from build123d import *

# Parameters (mm, degrees)
SKETCH1_W           = 5.08
SKETCH1_H           = 25.4
BOSS_EXTRUDE1_DEPTH = 5.08


with BuildPart() as part:
    # Sketch1 → Boss-Extrude1 (new body)
    with BuildSketch(Plane.XY):
        with BuildLine():
            Line((-13.447242614, 88.667051475), (-13.447242614, 93.747051475))
            Line((-13.447242614, 93.747051475), (9.557461427, 93.747051475))
            ThreePointArc((9.557461427, 93.747051475), (7.2409193, 101.644458486), (2.277698276, 108.209657797))
            Line((2.277698276, 108.209657797), (-45.487793081, 152.041039764))
            ThreePointArc((-45.487793081, 152.041039764), (-50.959133788, 159.684872704), (-52.891849255, 168.884240186))
            Line((-52.891849255, 168.884240186), (-52.891849255, 188.293861482))
            Line((-52.891849255, 188.293861482), (-52.891849255, 199.743466198))
            ThreePointArc((-52.891849255, 199.743466198), (-50.959133788, 208.94283368), (-45.487793081, 216.58666662))
            Line((-45.487793081, 216.58666662), (2.277698276, 260.418048586))
            ThreePointArc((2.277698276, 260.418048586), (7.2409193, 266.983247897), (9.557461427, 274.880654909))
            Line((9.557461427, 274.880654909), (-13.447242614, 274.880654909))
            Line((-13.447242614, 274.880654909), (-13.447242614, 279.960654909))
            Line((-13.447242614, 279.960654909), (-14.800406259, 279.960654909))
            Line((-14.800406259, 279.960654909), (-38.847242614, 279.960654909))
            Line((-38.847242614, 279.960654909), (-38.847242614, 274.880654909))
            Line((-38.847242614, 274.880654909), (-49.891849255, 274.880654909))
            Line((-49.891849255, 274.880654909), (-49.891849255, 264.914705614))
            Line((-49.891849255, 264.914705614), (-47.351849255, 264.914705614))
            Line((-47.351849255, 264.914705614), (-47.351849255, 262.414705614))
            Line((-47.351849255, 262.414705614), (-49.891849255, 262.414705614))
            Line((-49.891849255, 262.414705614), (-49.891849255, 260.680654909))
            Line((-49.891849255, 260.680654909), (-52.891849255, 260.680654909))
            Line((-52.891849255, 260.680654909), (-52.891849255, 262.414705614))
            Line((-52.891849255, 262.414705614), (-55.431849255, 262.414705614))
            Line((-55.431849255, 262.414705614), (-55.431849255, 264.914705614))
            Line((-55.431849255, 264.914705614), (-52.891849255, 264.914705614))
            Line((-52.891849255, 264.914705614), (-52.891849255, 274.880654909))
            Line((-52.891849255, 274.880654909), (-130.862222045, 274.880654909))
            Line((-130.862222045, 274.880654909), (-130.862222045, 264.914705614))
            Line((-130.862222045, 264.914705614), (-128.322222045, 264.914705614))
            Line((-128.322222045, 264.914705614), (-128.322222045, 262.414705614))
            Line((-128.322222045, 262.414705614), (-130.862222045, 262.414705614))
            Line((-130.862222045, 262.414705614), (-130.862222045, 260.680654909))
            Line((-130.862222045, 260.680654909), (-133.862222045, 260.680654909))
            Line((-133.862222045, 260.680654909), (-133.862222045, 262.414705614))
            Line((-133.862222045, 262.414705614), (-136.402222045, 262.414705614))
            Line((-136.402222045, 262.414705614), (-136.402222045, 264.914705614))
            Line((-136.402222045, 264.914705614), (-133.862222045, 264.914705614))
            Line((-133.862222045, 264.914705614), (-133.862222045, 274.880654909))
            Line((-133.862222045, 274.880654909), (-144.906828687, 274.880654909))
            Line((-144.906828687, 274.880654909), (-144.906828687, 279.960654909))
            Line((-144.906828687, 279.960654909), (-168.953665042, 279.960654909))
            Line((-168.953665042, 279.960654909), (-170.306828687, 279.960654909))
            Line((-170.306828687, 279.960654909), (-170.306828687, 274.880654909))
            Line((-170.306828687, 274.880654909), (-193.311532727, 274.880654909))
            ThreePointArc((-193.311532727, 274.880654909), (-190.9949906, 266.983247897), (-186.031769576, 260.418048586))
            Line((-186.031769576, 260.418048586), (-138.266278219, 216.58666662))
            ThreePointArc((-138.266278219, 216.58666662), (-132.794937512, 208.94283368), (-130.862222045, 199.743466198))
            Line((-130.862222045, 199.743466198), (-130.862222045, 188.293861482))
            Line((-130.862222045, 188.293861482), (-130.862222045, 168.884240186))
            ThreePointArc((-130.862222045, 168.884240186), (-132.794937512, 159.684872704), (-138.266278219, 152.041039764))
            Line((-138.266278219, 152.041039764), (-186.031769576, 108.209657797))
            ThreePointArc((-186.031769576, 108.209657797), (-190.9949906, 101.644458486), (-193.311532727, 93.747051475))
            Line((-193.311532727, 93.747051475), (-170.306828687, 93.747051475))
            Line((-170.306828687, 93.747051475), (-170.306828687, 88.667051475))
            Line((-170.306828687, 88.667051475), (-168.953665042, 88.667051475))
            Line((-168.953665042, 88.667051475), (-144.906828687, 88.667051475))
            Line((-144.906828687, 88.667051475), (-144.906828687, 93.747051475))
            Line((-144.906828687, 93.747051475), (-133.862222045, 93.747051475))
            Line((-133.862222045, 93.747051475), (-133.862222045, 103.713000769))
            Line((-133.862222045, 103.713000769), (-136.402222045, 103.713000769))
            Line((-136.402222045, 103.713000769), (-136.402222045, 106.213000769))
            Line((-136.402222045, 106.213000769), (-133.862222045, 106.213000769))
            Line((-133.862222045, 106.213000769), (-133.862222045, 107.947051475))
            Line((-133.862222045, 107.947051475), (-130.862222045, 107.947051475))
            Line((-130.862222045, 107.947051475), (-130.862222045, 106.213000769))
            Line((-130.862222045, 106.213000769), (-128.322222045, 106.213000769))
            Line((-128.322222045, 106.213000769), (-128.322222045, 103.713000769))
            Line((-128.322222045, 103.713000769), (-130.862222045, 103.713000769))
            Line((-130.862222045, 103.713000769), (-130.862222045, 93.747051475))
            Line((-130.862222045, 93.747051475), (-52.891849255, 93.747051475))
            Line((-52.891849255, 93.747051475), (-52.891849255, 103.713000769))
            Line((-52.891849255, 103.713000769), (-55.431849255, 103.713000769))
            Line((-55.431849255, 103.713000769), (-55.431849255, 106.213000769))
            Line((-55.431849255, 106.213000769), (-52.891849255, 106.213000769))
            Line((-52.891849255, 106.213000769), (-52.891849255, 107.947051475))
            Line((-52.891849255, 107.947051475), (-49.891849255, 107.947051475))
            Line((-49.891849255, 107.947051475), (-49.891849255, 106.213000769))
            Line((-49.891849255, 106.213000769), (-47.351849255, 106.213000769))
            Line((-47.351849255, 106.213000769), (-47.351849255, 103.713000769))
            Line((-47.351849255, 103.713000769), (-49.891849255, 103.713000769))
            Line((-49.891849255, 103.713000769), (-49.891849255, 93.747051475))
            Line((-49.891849255, 93.747051475), (-38.847242614, 93.747051475))
            Line((-38.847242614, 93.747051475), (-38.847242614, 88.667051475))
            Line((-38.847242614, 88.667051475), (-14.800406259, 88.667051475))
            Line((-14.800406259, 88.667051475), (-13.447242614, 88.667051475))
        make_face()
        with Locations((-91.87703565, 142.791515907)):
            Rectangle(SKETCH1_W, SKETCH1_H, mode=Mode.SUBTRACT)
        with Locations((-91.87703565, 233.796207057)):
            Rectangle(SKETCH1_W, SKETCH1_H, mode=Mode.SUBTRACT)
    extrude(amount=BOSS_EXTRUDE1_DEPTH)


solid = part.part
Check sheet for the modelled part. Datum: model origin and axes. Units: mm. A direction names the side the tool comes from. Give positions to 0.01 mm unless a question says otherwise; leave off trailing zeros. Write each loop counter-clockwise with the first axis right and the second up, starting at its lowest first coordinate (ties: lowest second). Pieces come first, ordered by that corner, then holes. Notation, with made-up numbers: (64.25, 83) -> (82.25, 83) arc R22 ccw to (82.25, 90) -> close; hole circle Ø2 at (-15.5, 64). An arc over 180 degrees is marked (long way). Write item = value, one per line.
Item 1: Sectioned sample at D-D on z = 1.05. Count the separate pieces of the cut face and the enclosed holes in it, and give its area (3 significant figures).
Output:
separate_pieces = 1
enclosed_holes = 2
area = 23,300 mm^2
Item 2: Sectioned sample at C-C on y = 100. Record the boundary of the cut face in (x, z), and give its area (3 significant figures).
Output:
outline = (-191.74, 0) -> (-133.86, 0) -> (-133.86, 5.08) -> (-191.74, 5.08) -> close; (-130.86, 0) -> (-52.89, 0) -> (-52.89, 5.08) -> (-130.86, 5.08) -> close; (-49.89, 0) -> (7.99, 0) -> (7.99, 5.08) -> (-49.89, 5.08) -> close
area = 984 mm^2
Item 3: Release check for a two-part mould opening along X. For faces 5 (the flat face through (-2, 274.881, 3)), 6 (the cylindrical face through (-132.74, 159.81, 2.5)), 7 (the flat face through (-49.892, 99, 3)), 8 (the flat face through (-92, 93.747, 3)) record: +X half, -X half, draft (parallel to the pull), parting line (faces both ways), or undercut.
Output:
face_5 = draft
face_6 = -X half
face_7 = undercut
face_8 = undercut
Item 4: Tool access check on faces 1 (the flat face through (-144.907, 91, 3)), 2 (the flat face through (-2, 93.747, 3)), 3 (the cylindrical face through (-190.94, 101.75, 2.5)), 4 (the flat face through (-52.892, 270, 3)). Record the directions out of +Z, -Z, +X, -X, +Y, -Y that give a thin tool (end or side, any length) a straight path to the whole face; none if there is none.
Output:
face_1 = +Z, -Z, -Y
face_2 = +Z, -Z, +X, -Y
face_3 = +Z, -Z, -X
face_4 = +Z, -Z, +Y
Item 5: Scan lines: probe 1 along Y at (x, z) = (-136, 4.45); probe 2 along X at (y, z) = (270, 1); probe 3 along X at (y, z) = (168.5, 3.25). Record each from-to range of solid material in increasing order. Write a range as from..to.
Output:
probe_1 = 93.75..103.71, 106.21..154.44, 214.18..262.41, 264.91..274.88
probe_2 = -192.25..-133.86, -130.86..-52.89, -49.89..8.5
probe_3 = -130.87..-52.89
Item 6: Gauge pin test, flat ends, axial feed: pin 1 (3 mm diameter, centred on x = -129, z = 1.5, fed in from -Y); pin 2 (1.5 mm diameter, centred on y = 228.5, z = 3, fed in from -X); pin 3 (0.9 mm diameter, centred on x = -132, z = 3, fed in from -Y). Record the tip position at first contact, or that the pin passes through.
Output:
pin_1 = 93.75
pin_2 = -152.07
pin_3 = 107.95
Item 7: Sectioned sample at A-A on y = 229.5. Record the boundary of the cut face in (x, z), and give its area (3 significant figures).
Output:
outline = (-152.34, 0) -> (-94.42, 0) -> (-94.42, 5.08) -> (-152.34, 5.08) -> close; (-89.34, 0) -> (-31.42, 0) -> (-31.42, 5.08) -> (-89.34, 5.08) -> close
area = 588 mm^2
Item 8: Sectioned sample at B-B on x = -158. Record the boundary of the cut face in (y, z), and give its area (3 significant figures).
Output:
outline = (88.67, 0) -> (133.93, 0) -> (133.93, 5.08) -> (88.67, 5.08) -> close; (234.7, 0) -> (279.96, 0) -> (279.96, 5.08) -> (234.7, 5.08) -> close
area = 460 mm^2
